```python
from build123d import *

# Parameters (mm, degrees)
BOSS_EXTRUDE2_DEPTH                      = 22
BOSS_EXTRUDE3_DEPTH                      = 10
FILLET1_R                                = 3
SKETCH3_R                                = 6
CUT_EXTRUDE1_DEPTH                       = 24
SKETCH4_R                                = 3
CUT_EXTRUDE2_DEPTH                       = 16
CBORE_START                              = 32
CBORE_FOR_M12_HEX_HEAD_BOLT3_OUTLINE_R   = 5
CBORE_FOR_M12_HEX_HEAD_BOLT3_DEPTH       = 4
CBORE_START_2                            = 25.196151292
CBORE_FOR_M12_HEX_HEAD_BOLT3_2_OUTLINE_R = 3
CBORE_FOR_M12_HEX_HEAD_BOLT3_2_DEPTH     = 6.803848708


# Read off the part's stored shape, not the designer's step: CBORE for M12 Hex Head Bolt3
with BuildPart() as part:
    # Sketch2 → Boss-Extrude2 (new body)
    with BuildSketch(Plane.XY):
        with BuildLine():
            Line((9.682876715, 10), (0, 10))
            Line((0, 10), (0, 0))
            Line((0, 0), (24, 0))
            Line((24, 0), (24, -9))
            Line((24, -9), (40, -9))
            Line((40, -9), (40, 0))
            Line((40, 0), (64, 0))
            Line((64, 0), (64, 10))
            Line((64, 10), (54.317123285, 10))
            Line((54.317123285, 10), (46.500924593, 26.761892188))
            ThreePointArc((46.500924593, 26.761892188), (32, 36), (17.499075407, 26.761892188))
            Line((17.499075407, 26.761892188), (9.682876715, 10))
        make_face()
    extrude(amount=BOSS_EXTRUDE2_DEPTH)

    # Sketch2<4> → Boss-Extrude3 (add)
    with BuildSketch(Plane.XY):
        Polygon((0, 0), (24, 0), (24, -9), (40, -9), (40, 0), (64, 0), (64, 36), (0, 36), align=None)
    extrude(amount=-BOSS_EXTRUDE3_DEPTH)

    # Fillet1
    fillet1_edges = [part.edges().sort_by_distance(p)[0] for p in [
        (54.317123285, 10, 11),
        (9.682876715, 10, 11),
    ]]
    fillet(fillet1_edges, radius=FILLET1_R)

    # Sketch3 → Cut-Extrude1 (cut)
    with BuildSketch(Plane.XY.offset(22)):
        with Locations((32, 20)):
            Circle(SKETCH3_R)
    extrude(amount=-CUT_EXTRUDE1_DEPTH, mode=Mode.SUBTRACT)

    # Sketch4 → Cut-Extrude2 (cut)
    with BuildSketch(Plane.XZ.offset(9)):
        with Locations((32, 14)):
            Circle(SKETCH4_R)
        with Locations((32, -2)):
            Circle(SKETCH4_R)
    extrude(amount=-CUT_EXTRUDE2_DEPTH, mode=Mode.SUBTRACT)

    # CBORE for M12 Hex Head Bolt3 outline → CBORE for M12 Hex Head Bolt3 (cut)
    with BuildSketch(Plane(origin=(0, 0, 0), x_dir=(1, 0, 0), z_dir=(0, 1, 0)).offset(CBORE_START)):
        with Locations((32, -10)):
            Circle(CBORE_FOR_M12_HEX_HEAD_BOLT3_OUTLINE_R)
    extrude(amount=CBORE_FOR_M12_HEX_HEAD_BOLT3_DEPTH, mode=Mode.SUBTRACT)

    # CBORE for M12 Hex Head Bolt3 2 outline → CBORE for M12 Hex Head Bolt3 2 (cut)
    with BuildSketch(Plane(origin=(0, 0, 0), x_dir=(1, 0, 0), z_dir=(0, 1, 0)).offset(CBORE_START_2)):
        with Locations((32, -10)):
            Circle(CBORE_FOR_M12_HEX_HEAD_BOLT3_2_OUTLINE_R)
    extrude(amount=CBORE_FOR_M12_HEX_HEAD_BOLT3_2_DEPTH, mode=Mode.SUBTRACT)


solid = part.part
```
Check sheet for the modelled part. Datum: model origin and axes. Units: mm. A direction names the side the tool comes from. Coordinates: 2 decimals unless noted, no trailing zeros. Order: outer loops, then holes, each group sorted by start corner. A loop starts at its lowest first (then second) coordinate and runs counter-clockwise, first axis right, second up. Notation, with made-up numbers: M 79,-8.75 L 135,-8.75 A7 ccw 135,1.25 Z; hole C -25.75,-36 d2. An arc over 180 degrees is marked long. Write each question's results on one line, items separated by ' | '. Start each with the question number.
1. Cross-section at A-A on z = 3.5. Record the cut outline in (x, y), and give its area (3 significant figures).
2. Cross-section at B-B on y = -1. Record the cut outline in (x, z).
3. Cross-section at D-D on z = 10. Record the cut outline in (x, y).
4. Access from +Z, -Z, +X, -X, +Y, -Y to the whole of each face (thin tool, end or side, straight path). Record for faces 1 (the face through (60, 10, 11)), 2 (the face through (9.4, 10.48, 11.15)), 3 (the face through (32, 20, -2)), 4 (the face through (29.6, -1.1, 12.2)), 5 (the face through (36.24, 35.43, 13.29)).
5. Go/stop test with flat-tipped pins: P1, Ø2.5, axis at y = -5, z = 12.5, coming from the -X side; P2, Ø12, axis at x = 51, z = 4.5, coming from the -Y side; P3, Ø8.5, axis at x = 60, z = 6, coming from the +Y side. Record where each tip stops, or that it passes through.
6. Cross-section at C-C on x = 59. Record the cut outline in (y, z).
7. Material ranges on probe 1 along Z at (x, y) = (32, 0.25); probe 2 along Z at (x, y) = (32, 28); probe 3 along Z at (x, y) = (32, 34.4), recorded low to high.
8. Mould release check, pull along Z, two halves, no side actions. Record for faces 6 (the face through (54.637, 10.457, 11.154)), 7 (the face through (31.9, 32, 13.3)), 8 (the face through (31.6, 13.8, 22)): +Z half, -Z half, draft (parallel to the pull), parting line (faces both ways), or undercut.
Checks:
1) outline: M 0,0 L 24,0 L 24,-9 L 40,-9 L 40,0 L 64,0 L 64,10 L 56.23,10 A3 cw 53.51,11.73 L 46.5,26.76 A16 ccw 17.5,26.76 L 10.49,11.73 A3 cw 7.77,10 L 0,10 Z; hole C 32,20 d12 | area: 1,480 mm²
2) outline: M 24,-10 L 40,-10 L 40,22 L 24,22 Z; hole C 32,-2 d6; hole C 32,14 d6
3) outline: M 0,0 L 24,0 L 24,-9 L 40,-9 L 40,0 L 64,0 L 64,10 L 56.23,10 A3 cw 53.51,11.73 L 46.5,26.76 A16 ccw 37,35.2 L 37,32 L 35,32 L 35,25.2 A6 cw long 29,25.2 L 29,32 L 27,32 L 27,35.2 A16 ccw 17.5,26.76 L 10.49,11.73 A3 cw 7.77,10 L 0,10 Z
4) face 1: +Z, +X, +Y | face 2: +Z, -X, +Y | face 3: +Z | face 4: -Y | face 5: +Z, +Y
5) P1: stops at x = 24 | P2: stops at y = 0 | P3: stops at y = 10.04
6) outline: M 0,-10 L 36,-10 L 36,0 L 10,0 L 10,22 L 0,22 Z
7) probe 1: z = -10 to -5, 1 to 11, 17 to 22 | probe 2: z = -10 to 7, 13 to 22 | probe 3: z = -10 to 5, 15 to 22
8) face 6: draft | face 7: undercut | face 8: +Z half
